Verification items for the finished model (mm, model axes). A direction names the side the tool comes from. Round coordinates to 2 decimals unless told otherwise and drop trailing zeros. Order: outer loops, then holes, each group sorted by start corner. A loop starts at its lowest first (then second) coordinate and runs counter-clockwise, first axis right, second up. Notation, with made-up numbers: M -20,28.25 L 38,28.25 A25 cw 38,59.25 Z; hole C 74,80.25 d7. An arc over 180 degrees is marked long. Use one line per item in the form item = value. Start each with the question number.
Item 1: Go/stop test with flat-tipped pins: pin 1 Ø8 at (x, y) = (-7, 22) entering from +Z; pin 2 Ø5 at (x, y) = (39, -4.5) entering from +Z; pin 3 Ø6 at (x, z) = (22.5, -59) entering from -Y. Record where each tip stops, or that it passes through.
Item 2: Cross-section at A-A on y = -12.7. Count the separate pieces of the cut face and the enclosed holes in it, then the cut area to 3 significant figures.
Item 3: Tool access check on faces 1 (the cylindrical face through (100.738, -12.842, -48.873)), 2 (the cylindrical face through (1.886, -11.406, -3.121)), 3 (the cylindrical face through (2.13, -15.08, 8.27)). Record the directions out of +Z, -Z, +X, -X, +Y, -Y that give a thin tool (end or side, any length) a straight path to the whole face; none if there is none.
Item 4: Cross-section at B-B on y = 12. Enter the section's corners in (x, z).
Item 5: Release check for a two-part mould opening along X. For faces 4 (the flat face through (41.865, -34.576, -56.148)), 5 (the flat face through (123, 32.11, -72)), 6 (the cylindrical face through (99.39, -11.41, -53.17)) record: +X half, -X half, draft (parallel to the pull), parting line (faces both ways), or undercut.
Item 6: Thickness scan on probe 1 along Y at (x, z) = (2, 0); probe 2 along Z at (x, y) = (25, 6.5); probe 3 along Z at (x, y) = (100, -2.5). Record the ranges inside material, lowest first. Write a range as [from, to].
from build123d import *

# Parameters (mm, degrees)
CUT_EXTRUDE1_DEPTH                                  = 198.511547075
CUT_EXTRUDE1_DEPTH_BACK                             = 198.511547075
CSK_FOR_1_4_FLAT_HEAD_MACHINE_SCREW_100_D           = 6.7564
CSK_FOR_1_4_FLAT_HEAD_MACHINE_SCREW_100_DEPTH       = 26.418979166
CSK_FOR_1_4_FLAT_HEAD_MACHINE_SCREW_100_CSINK_D     = 12.8778
CSK_FOR_1_4_FLAT_HEAD_MACHINE_SCREW_100_CSINK_ANGLE = 100
CIRPATTERN1_COUNT                                   = 3
FILLET1_R                                           = 25.4
SKETCH6_W                                           = 228.6
SKETCH6_H                                           = 42.39695855
CUT_EXTRUDE2_DEPTH                                  = 198.511547094
CUT_EXTRUDE2_DEPTH_BACK                             = 198.511547094


with BuildPart() as part:
    # Sketch2 → RevolvedVenturi-5inchOutsideDiaLower_2inchDeep (revolve)
    with BuildSketch(Plane.XY, mode=Mode.PRIVATE) as revolvedventuri_5inchoutsidedialower_2in_sk:
        with BuildLine():
            Line((0, 0), (1.5875, 0))
            Line((1.5875, 0), (1.5875, -38.1))
            Line((1.5875, -38.1), (4.7625, -38.1))
            Line((4.7625, -38.1), (4.7625, 0))
            ThreePointArc((4.7625, 0), (-4.071891712, 21.328108288), (-25.4, 30.1625))
            ThreePointArc((-25.4, 30.1625), (-35.487136871, 27.78125), (-25.4, 25.4))
            ThreePointArc((-25.4, 25.4), (-7.439487758, 17.960512242), (0, 0))
        make_face()
    revolve(revolvedventuri_5inchoutsidedialower_2in_sk.sketch.rotate(Axis((65.0875, -38.1, 0), (0, 1, 0)), 270), axis=Axis((65.0875, -38.1, 0), (0, 1, 0)))

    # Sketch3 → Cut-Extrude1 (cut, two sides)
    with BuildSketch(Plane.XY) as cut_extrude1_sk:
        Polygon((305.270582806, -11.53117295), (1.5875, -38.1), (5.893342851, -87.316008998), (309.576425657, -60.747181948), align=None)
    extrude(amount=CUT_EXTRUDE1_DEPTH, mode=Mode.SUBTRACT)
    extrude(cut_extrude1_sk.sketch, amount=-CUT_EXTRUDE1_DEPTH_BACK, mode=Mode.SUBTRACT)

    # CSK for 1/4 Flat Head Machine Screw (100)1
    with Locations(Plane(origin=(4.7625, -12.7, 0), x_dir=(0, 0, 1), z_dir=(1, 0, 0))):
        with Locations((0, 0)):
            csk_for_1_4_flat_head_machine_screw_100 = CounterSinkHole(CSK_FOR_1_4_FLAT_HEAD_MACHINE_SCREW_100_D / 2, CSK_FOR_1_4_FLAT_HEAD_MACHINE_SCREW_100_CSINK_D / 2, depth=CSK_FOR_1_4_FLAT_HEAD_MACHINE_SCREW_100_DEPTH, counter_sink_angle=CSK_FOR_1_4_FLAT_HEAD_MACHINE_SCREW_100_CSINK_ANGLE)

    # CirPattern1: CSK for 1/4 Flat Head Machine Screw (100)1 ×3 about axis
    cirpattern1_axis = Axis((65.0875, 0, 0), (0, -1, 0))
    for i in range(1, CIRPATTERN1_COUNT):
        add(csk_for_1_4_flat_head_machine_screw_100.rotate(cirpattern1_axis, i * 360 / CIRPATTERN1_COUNT), mode=Mode.SUBTRACT)

    # Fillet1
    fillet1_edges = [part.edges().sort_by_distance(p)[0] for p in [
        (65.0875, 30.1625, 90.4875),
    ]]
    fillet(fillet1_edges, radius=FILLET1_R)

    # Sketch6 → Cut-Extrude2 (cut, two sides)
    with BuildSketch(Plane.XY) as cut_extrude2_sk:
        with Locations((69.663229711, 53.30825)):
            Rectangle(SKETCH6_W, SKETCH6_H)
    extrude(amount=CUT_EXTRUDE2_DEPTH, mode=Mode.SUBTRACT)
    extrude(cut_extrude2_sk.sketch, amount=-CUT_EXTRUDE2_DEPTH_BACK, mode=Mode.SUBTRACT)


solid = part.part
Output values:
q1.pin_1 = 71.69
q1.pin_2 = 58.96
q1.pin_3 = 14.69
q2.separate_pieces = 3
q2.enclosed_holes = 0
q2.area = 1,140 mm2
q3.face_1 = none
q3.face_2 = -X
q3.face_3 = -Y
q4.outline = C 65.09,0 d136.2; hole C 65.09,0 d125.63
q5.face_4 = +X half
q5.face_5 = draft
q5.face_6 = undercut
q6.probe_1 = [-38.06, -16.08], [-9.32, 12.61]
q6.probe_2 = [-52.35, -46.02], [46.02, 52.35]
q6.probe_3 = [-53.04, -49.2], [49.2, 53.04]
